Check sheet for the modelled part. Datum: model origin and axes. Units: mm. Face numbers are marked on the shaded views. A direction names the side the tool comes from. Round coordinates to 2 decimals unless told otherwise and drop trailing zeros. Order: outer loops, then holes, each group sorted by start corner. A loop starts at its lowest first (then second) coordinate and runs counter-clockwise, first axis right, second up.
Q1. Cross-section at A-A on y = 6.5. Record the cut outline in (x, z), then the cut area to 3 significant figures.
Q2. Scan lines: probe 1 along Y at (x, z) = (-21.75, 0); probe 2 along Y at (x, z) = (-20, 0); probe 3 along Z at (x, y) = (21.75, 6.5). Record each from-to range of solid material in increasing order.
Q3. Cross-section at B-B on y = 20. Record the cut outline in (x, z), then the cut area to 3 significant figures.
Q4. Mould release check, pull along Y, two halves, no side actions. Record for the marked faces 1 and 2: +Y half, -Y half, draft (parallel to the pull), parting line (faces both ways), or undercut.
Q5. Set-up check for the marked faces 3 and 4: record each of +Z, -Z, +X, -X, +Y, -Y from which the full face is reachable in a straight line by a thin tool's end or side.
Q6. Depth check by flat-ended pin: P1, Ø0.5, axis at x = 5, y = 0.5, coming from the +Z side; P2, Ø1.1, axis at x = 2.5, y = 0.5, coming from the +Z side; P3, Ø1.5, axis at y = 8, z = -19.5, coming from the +X side. Enter the tip coordinate at first touch or a pass-through.
Autodesk Fusion 360 part; units mm, degrees
sketch "Sketch1" plane through (0, 0, 0) normal (0, 1, 0) x (1, 0, 0)
  circle A0 centre (0, 0) radius 27.5
  dimension "d1" = 55
extrude "Extrude1" add sketch "Sketch1" along normal blind 4
sketch "Sketch2" plane through (0, 4, 0) normal (0, 1, 0) x (-1, 0, 0)
  circle A0 centre (0, 0) radius 27.5
  circle A1 centre (0, 0) radius 25.3
  dimension "d4" = 50.6
extrude "Extrude2" add sketch "Sketch2" along normal blind 5 contours A1
sketch "Sketch3" plane through (0, 0, 0) normal (0, -1, 0) x (1, 0, 0)
  circle A0 centre (0, 0) radius 27.5
  line L0 (21.5985, 0) -> (19.1914, -4.1689)
  line L1 (3.5784, -14.5357) -> (-13.1761, -14.5877)
  line L2 (-11.9706, 0) -> (-14.3773, 4.1693)
  line L3 (-14.3773, 4.1693) -> (-5.9851, -10.3664)
  line L4 (14.3777, -4.1689) -> (6.0451, -18.7046)
  line L5 (5.9851, -10.3664) -> (3.5784, -14.5357)
  line L6 (-14.3773, 4.1693) -> (-6.0451, 18.705)
  line L7 (-5.9851, 18.705) -> (-14.3773, 4.1693)
  line L8 (-10.7992, -10.3664) -> (-19.2216, 4.1173)
  line L9 (-19.1914, 4.1693) -> (-10.7992, -10.3664)
  line L10 (-10.7992, -18.7046) -> (-13.2063, -14.5357)
  line L11 (-5.9851, -10.3664) -> (-10.7992, -10.3664)
  line L12 (-21.5985, 0) -> (-19.1914, 4.1693)
  line L13 (10.7992, 10.3668) -> (19.2216, -4.1169)
  line L14 (-10.7992, -10.3664) -> (5.9851, -10.3664)
  line L15 (-13.2063, -14.5357) -> (3.5784, -14.5357)
  line L16 (14.3777, -4.1689) -> (5.9851, 10.3668)
  line L17 (13.2063, 14.5357) -> (-3.578, 14.5357)
  line L18 (6.0451, -18.7046) -> (-10.7992, -18.7046)
  line L19 (11.9706, 0) -> (14.3777, -4.1689)
  line L20 (19.1914, -4.1689) -> (10.7992, 10.3668)
  line L21 (5.9851, -18.7046) -> (14.3777, -4.1689)
  line L22 (13.1765, 14.5877) -> (21.5985, 0)
  line L23 (-6.0451, 18.705) -> (10.7992, 18.705)
  line L24 (-3.578, 14.5357) -> (-11.9706, 0)
  line L25 (10.7992, 10.3668) -> (-5.9851, 10.3668)
  line L26 (10.7992, -18.7046) -> (5.9851, -18.7046)
  line L27 (19.2216, -4.1169) -> (10.7992, -18.7046)
  line L28 (10.7992, 18.705) -> (13.2063, 14.5357)
  line L29 (-11.9706, 0) -> (11.9706, 0)
  line L30 (0, 0) -> (0, 10.3668)
  line L31 (-19.2216, 4.1173) -> (-10.7992, 18.705)
  line L32 (-13.1761, -14.5877) -> (-21.5985, 0)
  line L33 (-10.7992, 18.705) -> (-5.9851, 18.705)
  line L34 (3.5784, -14.5357) -> (11.9706, 0)
  line L35 (5.9851, 10.3668) -> (10.7992, 10.3668)
  line L36 (-3.578, 14.5357) -> (13.1765, 14.5877)
  line L37 (-5.9851, 10.3668) -> (-3.578, 14.5357)
  line L38 (-13.2236, 4.171) -> (-5.4656, 17.705)
  line L39 (-5.4656, 17.705) -> (10.2219, 17.705)
  line L40 (10.2219, 17.705) -> (11.4743, 15.5357)
  line L41 (11.4743, 15.5357) -> (-4.1554, 15.5357)
  line L42 (-4.1554, 15.5357) -> (-11.9705, 2.0001)
  line L43 (-11.9705, 2.0001) -> (-13.2236, 4.171)
  line L44 (11.3766, 11.3668) -> (-4.253, 11.3668)
  line L45 (-4.253, 11.3668) -> (-2.9997, 13.5375)
  line L46 (-2.9997, 13.5375) -> (12.6002, 13.5859)
  line L47 (12.6002, 13.5859) -> (20.4438, 0)
  line L48 (20.4438, 0) -> (19.1914, -2.1689)
  line L49 (19.1914, -2.1689) -> (11.3766, 11.3668)
  line L50 (10.224, 9.3668) -> (18.0659, -4.1187)
  line L51 (18.0659, -4.1187) -> (10.2219, -17.7046)
  line L52 (10.2219, -17.7046) -> (7.7172, -17.7046)
  line L53 (7.7172, -17.7046) -> (15.5324, -4.1689)
  line L54 (15.5324, -4.1689) -> (7.7172, 9.3668)
  line L55 (7.7172, 9.3668) -> (10.224, 9.3668)
  line L56 (13.224, -4.1707) -> (5.4657, -17.7046)
  line L57 (5.4657, -17.7046) -> (-10.2219, -17.7046)
  line L58 (-10.2219, -17.7046) -> (-11.4742, -15.5357)
  line L59 (-11.4742, -15.5357) -> (4.1558, -15.5357)
  line L60 (4.1558, -15.5357) -> (11.9706, -2)
  line L61 (11.9706, -2) -> (13.224, -4.1707)
  line L62 (3, -13.5375) -> (-12.5998, -13.5859)
  line L63 (-12.5998, -13.5859) -> (-20.4438, 0)
  line L64 (-20.4438, 0) -> (-19.1914, 2.1693)
  line L65 (-19.1914, 2.1693) -> (-11.3766, -11.3664)
  line L66 (-11.3766, -11.3664) -> (4.2532, -11.3664)
  line L67 (4.2532, -11.3664) -> (3, -13.5375)
  line L68 (-10.224, -9.3664) -> (-18.0659, 4.1191)
  line L69 (-18.0659, 4.1191) -> (-10.2219, 17.705)
  line L70 (-10.2219, 17.705) -> (-7.7172, 17.705)
  line L71 (-7.7172, 17.705) -> (-15.532, 4.1693)
  line L72 (-15.532, 4.1693) -> (-7.7172, -9.3664)
  line L73 (-7.7172, -9.3664) -> (-10.224, -9.3664)
  dimension "d8" = 1
  dimension "d9" = 1
  dimension "d10" = 1
  dimension "d11" = 1
  dimension "d12" = 1
  dimension "d13" = 1
extrude "Extrude3" cut sketch "Sketch3" against normal blind 1 contours L38 L39 L40 L41 L42 L43 | L44 L45 L46 L47 L48 L49 | L50 L51 L52 L53 L54 L55 | L56 L57 L58 L59 L60 L61 | L62 L63 L64 L65 L66 L67 | L68 L69 L70 L71 L72 L73
chamfer "Chamfer1" distance 2 angle 45 1 edges at (-25.639, 0, 9.9444)
sketch "Sketch5" plane through (0, 0, 0) normal (0, 0, 1) x (1, 0, 0)
  line L0 (25.3, 9) -> (-25.3, 9)
  line L1 (25.3, 9) -> (0, 26.7153)
  line L2 (25.3, 9) -> (54.9449, 9) construction
  line L3 (0, 26.7153) -> (0, 9)
  line L4 (0, 26.7153) -> (0, 24.5)
  dimension "d19" = 145
  dimension "d37" = 30.8856
revolve "Revolve1" add sketch "Sketch5" angle 360 about axis through (0, 1.75, 0) along (0, 1, 0)
ref_plane "WorkPlane3" through (25.3, 0, 0) normal (1, 0, 0) x (0, 1, 0)
sketch "Sketch8" plane through (25.3, 0, 0) normal (1, 0, 0) x (0, 0, -1)
  line L0 (0, 9) -> (0, 6.5)
  circle A0 centre (0, 6.5) radius 1.4
  point P0 (0, 9)
  dimension "d28" = 2.5
  dimension "d29" = 2.8
extrude "Extrude6" cut sketch "Sketch8" against normal blind 8
ref_plane "WorkPlane4" through (-25.3, 0, 0) normal (1, 0, 0) x (0, 1, 0)
sketch "Sketch9" plane through (-25.3, 0, 0) normal (1, 0, 0) x (0, 0, -1)
  line L0 (0, 9) -> (0, 6.5)
  circle A0 centre (0, 6.5) radius 1.4
  point P0 (0, 9)
  dimension "d33" = 2.5
  dimension "d34" = 2.8
extrude "Extrude7" cut sketch "Sketch9" along normal blind 8
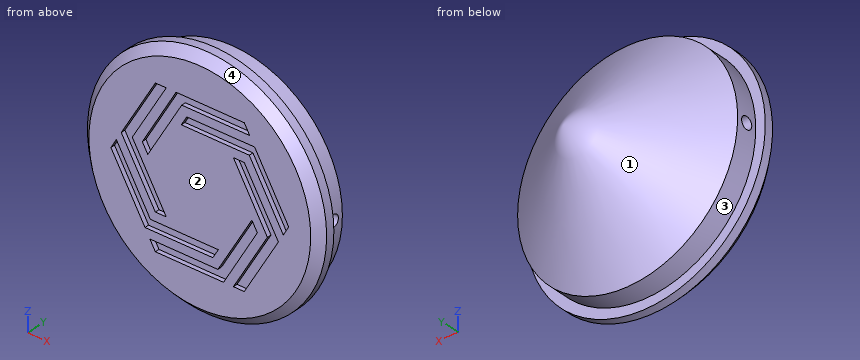
Results found:
1. outline: (-25.26, -1.4) arc R25.3 ccw to (25.26, -1.4) - (17.3, -1.4) - (17.3, 1.4) - (25.26, 1.4) arc R25.3 ccw to (-25.26, 1.4) - (-17.3, 1.4) - (-17.3, -1.4) - close
1. area: 1,970 mm2
2. probe 1: y = 0 to 5.1, 7.9 to 11.49
2. probe 2: y = 1 to 5.1, 7.9 to 12.71
2. probe 3: z = -12.92 to -1.4, 1.4 to 12.92
3. outline: circle Ø19.18 at (0, 0)
3. area: 289 mm2
4. face 1: +Y half
4. face 2: -Y half
5. face 3: +Y
5. face 4: -Y
6. P1: stops at z = 25.77
6. P2: stops at z = 26.43
6. P3: stops at x = 16.99
